Answer from the drawing. Dimensions are ordinates in mm from the lowest x, y and z of the part. Round coordinates to 2 decimals unless told otherwise and drop trailing zeros. Loops run counter-clockwise (first coordinate to the right, second up) from the corner with the lowest first, then second, coordinate; pieces in that order, holes last.
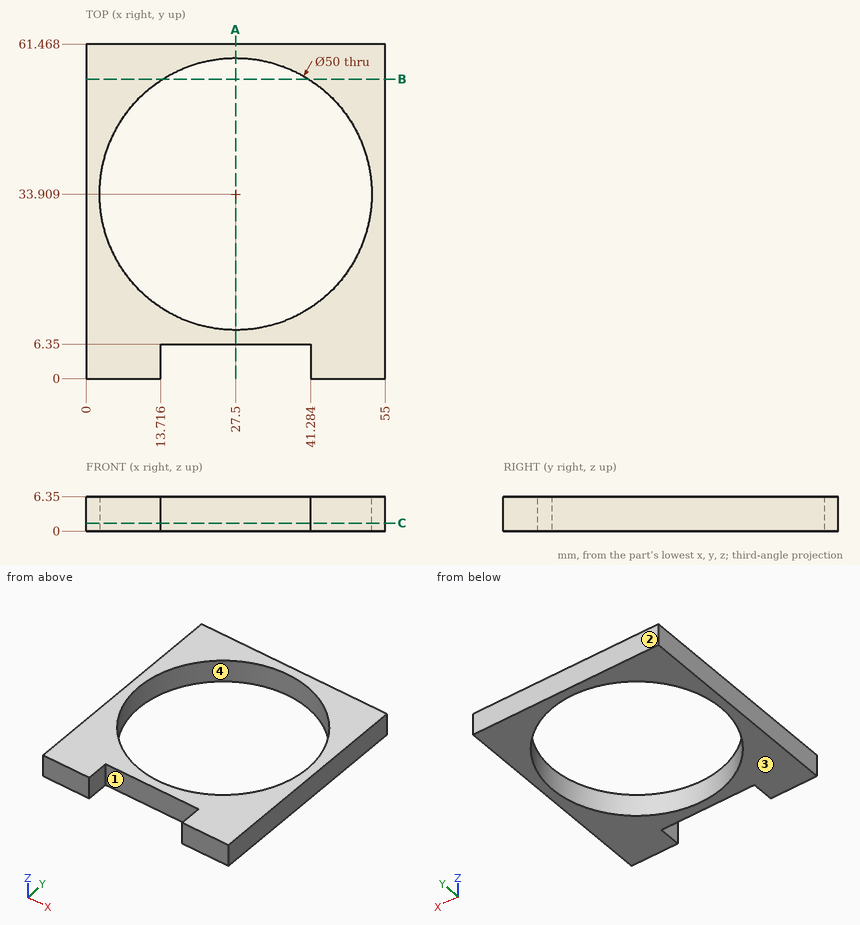
Item 1: Section C-C, the plane z = 1.5 is taken. Give the vertices of the cut face in (x, y), plus the area to 3 significant figures.
Item 2: Determine the mould class of the marked faces 1, 2, 3 and 4 for opening direction Y: pulls with the +Y half, pulls with the -Y half, needs draft (parallel to the pull), parting line crosses it, or undercut.
Item 3: Section B-B, the plane y = 55 is taken. Give the vertices of the cut face in (x, z).
Item 4: Each of these flat-tipped pins is pushed along its axis until it touches: P1, Ø3, axis at x = 40, z = 2.5, coming from the -Y side; P2, Ø3, axis at x = 24.5, z = 3, coming from the -Y side. Where does it stop, or does it pass through?
Item 5: Section A-A, the plane x = 27.5 is taken. Give the vertices of the cut face in (y, z).
Item 6: Straight lines are drawn through the part: line 1 (Y direction, x = 27.5, z = 4.75); line 2 (X direction, y = 24, z = 5.5); line 3 (Y direction, x = 49.5, z = 2.5). For each, find the intervals that lie inside material, in ascending order.
Answer below:
1. outline: (0, 0) - (13.72, 0) - (13.72, 6.35) - (41.28, 6.35) - (41.28, 0) - (55, 0) - (55, 61.47) - (0, 61.47) - close; hole circle Ø50 at (27.5, 33.91)
1. area: 1,240 mm2
2. face 1: pulls with the -Y half
2. face 2: pulls with the +Y half
2. face 3: needs draft
2. face 4: undercut
3. outline: (0, 0) - (14.08, 0) - (14.08, 6.35) - (0, 6.35) - close; (40.92, 0) - (55, 0) - (55, 6.35) - (40.92, 6.35) - close
4. P1: stops at y = 0
4. P2: stops at y = 6.35
5. outline: (6.35, 0) - (8.91, 0) - (8.91, 6.35) - (6.35, 6.35) - close; (58.91, 0) - (61.47, 0) - (61.47, 6.35) - (58.91, 6.35) - close
6. line 1: y = 6.35 to 8.91, 58.91 to 61.47
6. line 2: x = 0 to 4.55, 50.45 to 55
6. line 3: y = 0 to 22.03, 45.78 to 61.47
